Geometry: see drawing. Coordinates: mm, zero at the bounding-box minimum. A direction names the side the tool comes from. Coordinates: 2 decimals unless noted, no trailing zeros. Write each loop counter-clockwise with the first axis right and the second up, starting at its lowest first coordinate (ties: lowest second). Pieces come first, ordered by that corner, then holes. Notation, with made-up numbers: M 87.5,40 L 121.5,40 A20 ccw 121.5,55 Z; hole C 78.5,42.25 d4. An arc over 180 degrees is marked long. Write item = value, one per line. Start each with the question number.
1. Section query A-A (x = 12.5). Output: boundary loops of the cut face in (y, z), then the cut area to 3 significant figures.
2. Section query D-D (y = 20.25). Output: boundary loops of the cut face in (x, z).
3. Pin query (flat end, axial travel): pin 1 Ø4 at (x, z) = (25, 31) entering from +Y; pin 2 Ø1.2 at (x, y) = (35.5, 2.5) entering from +Z; pin 3 Ø1.2 at (y, z) = (2, 54) entering from +X. Return the tip coordinate at first contact, or that it passes through.
4. Line query: line 1 along X through (y, z) = (1.95, 77.5); line 2 along Y through (x, z) = (36, 2.15); line 3 along Y through (x, z) = (39, 21.5). Output: solid intervals per line, ascending.
5. Access query for the marked faces 1 and 2. Directions: +Z, -Z, +X, -X, +Y, -Y. A direction counts if a zero-diameter tool reaches every point of the face in a straight line with its end or side. Return the directions, or none.
6. Section query B-B (z = 18.5). Output: boundary loops of the cut face in (x, y).
7. Section query C-C (x = 33.5). Output: boundary loops of the cut face in (y, z).
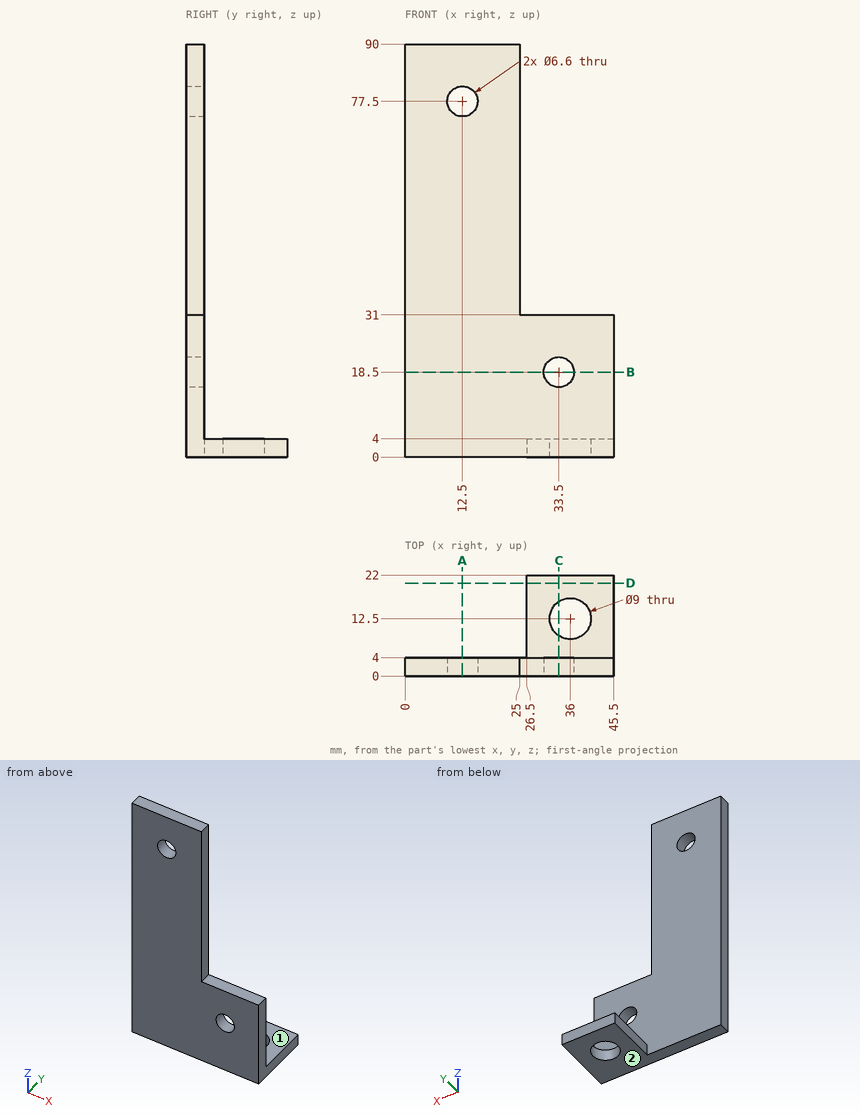
Results are:
q1.outline = M 0,0 L 4,0 L 4,74.2 L 0,74.2 Z; M 0,80.8 L 4,80.8 L 4,90 L 0,90 Z
q1.area = 334 mm^2
q2.outline = M 26.5,0 L 45.5,0 L 45.5,4 L 26.5,4 Z
q3.pin_1 = 4
q3.pin_2 = 31
q3.pin_3 = 25
q4.line_1 = 0 to 9.2, 15.8 to 25
q4.line_2 = 0 to 8, 17 to 22
q4.line_3 = 0 to 4
q5.face_1 = +Z, +X, -X, +Y
q5.face_2 = -Z, +X, -X, +Y, -Y
q6.outline = M 0,0 L 30.2,0 L 30.2,4 L 0,4 Z; M 36.8,0 L 45.5,0 L 45.5,4 L 36.8,4 Z
q7.outline = M 0,0 L 8.76,0 L 8.76,4 L 4,4 L 4,15.2 L 0,15.2 Z; M 0,21.8 L 4,21.8 L 4,31 L 0,31 Z; M 16.24,0 L 22,0 L 22,4 L 16.24,4 Z
